from build123d import *
from build123d.topology import SkipClean

# Parameters (mm, degrees)
SKETCH1_R            = 50.8
SKETCH1_W            = 25.4
SKETCH1_H            = 31.75
BOSS_EXTRUDE3_DEPTH  = 50.8
SKETCH2_R            = 50.8
BOSS_EXTRUDE4_DEPTH  = 27.94
SKETCH3_R            = 50.8
BOSS_EXTRUDE5_DEPTH  = 50.8
SKETCH4_R            = 50.8
BOSS_EXTRUDE6_DEPTH  = 27.94
SKETCH5_R            = 50.8
SKETCH5_W            = 25.4
SKETCH5_H            = 31.75
BOSS_EXTRUDE7_DEPTH  = 27.94
BOSS_EXTRUDE8_START  = 27.94
SKETCH6_R            = 50.8
BOSS_EXTRUDE8_DEPTH  = 27.94
BOSS_EXTRUDE9_START  = 50.8
SKETCH7_R            = 50.8
SKETCH7_W            = 31.75
SKETCH7_H            = 25.4
BOSS_EXTRUDE9_DEPTH  = 50.8
BOSS_EXTRUDE10_START = 27.94
SKETCH8_R            = 50.8
BOSS_EXTRUDE10_DEPTH = 27.94
BOSS_EXTRUDE11_START = 27.94
SKETCH9_R            = 50.8
SKETCH9_W            = 25.4
SKETCH9_H            = 31.75
BOSS_EXTRUDE11_DEPTH = 27.94
SKETCH10_R           = 50.8
BOSS_EXTRUDE12_DEPTH = 8.89
BOSS_EXTRUDE13_START = 8.89
SKETCH11_R           = 50.8
BOSS_EXTRUDE13_DEPTH = 8.89
SKETCH12_R           = 25.4
BOSS_EXTRUDE14_DEPTH = 8.89
BOSS_EXTRUDE15_START = 8.89
SKETCH13_R           = 25.4
BOSS_EXTRUDE15_DEPTH = 8.89
SKETCH14_R           = 5
CUT_EXTRUDE1_DEPTH   = 369.166294367
CHAMFER3_SIZE        = 8.89


with BuildPart() as part:
    # Sketch1 → Boss-Extrude3 (new body)
    with BuildSketch(Plane(origin=(0, 0, 0), x_dir=(0, 0, -1), z_dir=(1, 0, 0))):
        Circle(SKETCH1_R)
        with Locations((0, 50.8)):
            Rectangle(SKETCH1_W, SKETCH1_H)
        Polygon((51.392243797, 44.336022628), (23.895937227, 28.461022628), (36.595937227, 6.463977372), (64.092243797, 22.338977372), align=None)
        Polygon((64.092243797, -22.338977372), (36.595937227, -6.463977372), (23.895937227, -28.461022628), (51.392243797, -44.336022628), align=None)
        with Locations((0, -50.8)):
            Rectangle(SKETCH1_W, SKETCH1_H)
        Polygon((-51.392243797, -44.336022628), (-23.895937227, -28.461022628), (-36.595937227, -6.463977372), (-64.092243797, -22.338977372), align=None)
        Polygon((-64.092243797, 22.338977372), (-36.595937227, 6.463977372), (-23.895937227, 28.461022628), (-51.392243797, 44.336022628), align=None)
    extrude(amount=BOSS_EXTRUDE3_DEPTH)

    # Sketch2 → Boss-Extrude4 (add)
    with BuildSketch(Plane(origin=(50.8, 0, 0), x_dir=(0, 0, -1), z_dir=(1, 0, 0))):
        with Locations(Location((0, 0, 0), (0, 0, 164.477512186))):
            Circle(SKETCH2_R)
    extrude(amount=BOSS_EXTRUDE4_DEPTH)

    # Sketch3 → Boss-Extrude5 (add)
    with BuildSketch(Plane(origin=(78.74, 0, 0), x_dir=(0, 0, -1), z_dir=(1, 0, 0))):
        with Locations(Location((0, 0, 0), (0, 0, 165.522487814))):
            Circle(SKETCH3_R)
        Polygon((36.437276545, 12.7), (36.437276545, 0), (36.437276545, -12.7), (68.187276545, -12.7), (68.187276545, 12.7), align=None)
        Polygon((18.218638272, 31.555607132), (29.2171609, 25.205607132), (45.0921609, 52.701913703), (23.095115644, 65.401913703), (7.220115644, 37.905607132), align=None)
        Polygon((29.2171609, -25.205607132), (18.218638272, -31.555607132), (7.220115644, -37.905607132), (23.095115644, -65.401913703), (45.0921609, -52.701913703), align=None)
        Polygon((-7.220115644, -37.905607132), (-18.218638272, -31.555607132), (-29.2171609, -25.205607132), (-45.0921609, -52.701913703), (-23.095115644, -65.401913703), align=None)
        Polygon((-36.437276545, -12.7), (-36.437276545, 0), (-36.437276545, 12.7), (-68.187276545, 12.7), (-68.187276545, -12.7), align=None)
        Polygon((-29.2171609, 25.205607132), (-18.218638272, 31.555607132), (-7.220115644, 37.905607132), (-23.095115644, 65.401913703), (-45.0921609, 52.701913703), align=None)
    extrude(amount=BOSS_EXTRUDE5_DEPTH)

    # Sketch4 → Boss-Extrude6 (add)
    with BuildSketch(Plane(origin=(129.54, 0, 0), x_dir=(0, 0, -1), z_dir=(1, 0, 0))):
        with Locations(Location((0, 0, 0), (0, 0, 164.477512186))):
            Circle(SKETCH4_R)
    extrude(amount=BOSS_EXTRUDE6_DEPTH)

    # Sketch5 → Boss-Extrude7 (add)
    with BuildSketch(Plane(origin=(157.48, 0, 0), x_dir=(0, 0, -1), z_dir=(1, 0, 0))):
        with Locations(Location((0, 0, 0), (0, 0, 164.477512186))):
            Circle(SKETCH5_R)
        with Locations((0, 50.8)):
            Rectangle(SKETCH5_W, SKETCH5_H)
        Polygon((51.392243797, 44.336022628), (23.895937227, 28.461022628), (36.595937227, 6.463977372), (64.092243797, 22.338977372), align=None)
        Polygon((64.092243797, -22.338977372), (36.595937227, -6.463977372), (23.895937227, -28.461022628), (51.392243797, -44.336022628), align=None)
        with Locations((0, -50.8)):
            Rectangle(SKETCH5_W, SKETCH5_H)
        Polygon((-51.392243797, -44.336022628), (-23.895937227, -28.461022628), (-36.595937227, -6.463977372), (-64.092243797, -22.338977372), align=None)
        Polygon((-64.092243797, 22.338977372), (-36.595937227, 6.463977372), (-23.895937227, 28.461022628), (-51.392243797, 44.336022628), align=None)
    extrude(amount=BOSS_EXTRUDE7_DEPTH)

    # Sketch6 → Boss-Extrude8 (add)
    with SkipClean():  # the faces are left unmerged after this step: merging them gives an invalid solid
        with BuildSketch(Plane.ZY.offset(BOSS_EXTRUDE8_START)):
            Circle(SKETCH6_R)
        extrude(amount=-BOSS_EXTRUDE8_DEPTH)

    # Sketch7 → Boss-Extrude9 (add)
    with SkipClean():  # the faces are left unmerged after this step: merging them gives an invalid solid
        with BuildSketch(Plane.ZY.offset(27.94).offset(BOSS_EXTRUDE9_START)):
            with Locations(Location((0, 0, 0), (0, 0, 345.522487814))):
                Circle(SKETCH7_R)
            Polygon((23.095115644, 65.401913703), (45.0921609, 52.701913703), (29.2171609, 25.205607132), (7.220115644, 37.905607132), align=None)
            with Locations((52.312276545, 0)):
                Rectangle(SKETCH7_W, SKETCH7_H)
            Polygon((29.2171609, -25.205607132), (45.0921609, -52.701913703), (23.095115644, -65.401913703), (7.220115644, -37.905607132), align=None)
            Polygon((-7.220115644, -37.905607132), (-23.095115644, -65.401913703), (-45.0921609, -52.701913703), (-29.2171609, -25.205607132), align=None)
            with Locations((-52.312276545, 0)):
                Rectangle(SKETCH7_W, SKETCH7_H)
            Polygon((-29.2171609, 25.205607132), (-45.0921609, 52.701913703), (-23.095115644, 65.401913703), (-7.220115644, 37.905607132), align=None)
        extrude(amount=-BOSS_EXTRUDE9_DEPTH)

    # Sketch8 → Boss-Extrude10 (add)
    with SkipClean():  # the faces are left unmerged after this step: merging them gives an invalid solid
        with BuildSketch(Plane.ZY.offset(78.74).offset(BOSS_EXTRUDE10_START)):
            Circle(SKETCH8_R)
        extrude(amount=-BOSS_EXTRUDE10_DEPTH)

    # Sketch9 → Boss-Extrude11 (add)
    with SkipClean():  # the faces are left unmerged after this step: merging them gives an invalid solid
        with BuildSketch(Plane.ZY.offset(106.68).offset(BOSS_EXTRUDE11_START)):
            with Locations(Location((0, 0, 0), (0, 0, 15.522487814))):
                Circle(SKETCH9_R)
            with Locations((0, 50.8)):
                Rectangle(SKETCH9_W, SKETCH9_H)
            Polygon((51.392243797, 44.336022628), (23.895937227, 28.461022628), (36.595937227, 6.463977372), (64.092243797, 22.338977372), align=None)
            Polygon((64.092243797, -22.338977372), (36.595937227, -6.463977372), (23.895937227, -28.461022628), (51.392243797, -44.336022628), align=None)
            with Locations((0, -50.8)):
                Rectangle(SKETCH9_W, SKETCH9_H)
            Polygon((-51.392243797, -44.336022628), (-23.895937227, -28.461022628), (-36.595937227, -6.463977372), (-64.092243797, -22.338977372), align=None)
            Polygon((-64.092243797, 22.338977372), (-36.595937227, 6.463977372), (-23.895937227, 28.461022628), (-51.392243797, 44.336022628), align=None)
        extrude(amount=-BOSS_EXTRUDE11_DEPTH)

    # Sketch10 → Boss-Extrude12 (add)
    with SkipClean():  # the faces are left unmerged after this step: merging them gives an invalid solid
        with BuildSketch(Plane(origin=(185.42, 0, 0), x_dir=(0, 0, -1), z_dir=(1, 0, 0))):
            with Locations(Location((0, 0, 0), (0, 0, 195.522487814))):
                Circle(SKETCH10_R)
        extrude(amount=BOSS_EXTRUDE12_DEPTH)

    # Sketch11 → Boss-Extrude13 (add)
    with SkipClean():  # the faces are left unmerged after this step: merging them gives an invalid solid
        with BuildSketch(Plane.ZY.offset(134.62).offset(BOSS_EXTRUDE13_START)):
            Circle(SKETCH11_R)
        extrude(amount=-BOSS_EXTRUDE13_DEPTH)

    # Sketch12 → Boss-Extrude14 (add)
    with SkipClean():  # the faces are left unmerged after this step: merging them gives an invalid solid
        with BuildSketch(Plane(origin=(194.31, 0, 0), x_dir=(0, 0, -1), z_dir=(1, 0, 0))):
            Circle(SKETCH12_R)
        extrude(amount=BOSS_EXTRUDE14_DEPTH)

    # Sketch13 → Boss-Extrude15 (add)
    with SkipClean():  # the faces are left unmerged after this step: merging them gives an invalid solid
        with BuildSketch(Plane.ZY.offset(143.51).offset(BOSS_EXTRUDE15_START)):
            with Locations(Location((0, 0, 0), (0, 0, 180))):
                Circle(SKETCH13_R)
        extrude(amount=-BOSS_EXTRUDE15_DEPTH)

    # Sketch14 → Cut-Extrude1 (cut, through all)
    with SkipClean():  # the faces are left unmerged after this step: merging them gives an invalid solid
        with BuildSketch(Plane.ZY.offset(152.4)):
            Circle(SKETCH14_R)
        extrude(amount=-CUT_EXTRUDE1_DEPTH, mode=Mode.SUBTRACT)

    # Chamfer3
    chamfer3_edges = [part.edges().sort_by_distance(p)[0] for p in [
        (194.31, 0, 25.4),
        (-143.51, 0, 25.4),
    ]]
    chamfer(chamfer3_edges, length=CHAMFER3_SIZE - 0.0001)  # a hair under: the kernel refuses the full size


solid = part.part
Input: part model. Units: mm. Frame: model coordinates. A direction names the side the tool comes from. Coordinates: 2 decimals unless noted, no trailing zeros. Order: outer loops, then holes, each group sorted by start corner. A loop starts at its lowest first (then second) coordinate and runs counter-clockwise, first axis right, second up. Notation, with made-up numbers: M 74,11.25 L 114,11.25 A14 ccw 114,21.25 Z; hole C -33,74 d11. An arc over 180 degrees is marked long. Write item = value, one per line. Start each with the question number.
(1) First-contact query: P1, Ø1.5, axis at y = 25.5, z = 1.5, coming from the -X side; P2, Ø5, axis at x = 38, y = -31, coming from the +Z side; P3, Ø5.5, axis at y = 3, z = 58.5, coming from the +X side; P4, Ø1.5, axis at x = 51.5, y = 46.5, coming from the +Z side. Flat tips, straight axial feed; report the tip coordinate or a pass-through.
(2) Reachability of faces 1 (the flat face through (104, -12.7, 59)), 2 (the flat face through (104, -12.7, -59)), 3 (the flat face through (194.31, 29, 19)), 4 (the flat face through (0, 29, -50)) from +Z, -Z, +X, -X, +Y, -Y: full face, straight path, thin tool, end or side. Return the list, or none.
(3) Pull-direction query (Y, two-part tool) for faces 5 (the flat face through (25.04, -18.03, -56.63)), 6 (the flat face through (185.42, -29, 50)), 7 (the flat face through (25, -66.675, 0)); classes: released by +Y, released by -Y, zero draft, split by the parting line, or undercut.
(4) Section B-B on x = -62. Output: boundary loops of the cut face in (y, z).
(5) Section C-C on y = -40. Give the number of separate pieces and of enclosed holes in the cut face, and give its area (3 significant figures).
(6) Line query: line 1 along X through (y, z) = (-39, 52); line 2 along Y through (x, z) = (121.5, 0); line 3 along Y through (x, z) = (46, 0) (3 decimals). Output: solid intervals per line, ascending. Write a range as [from, to].
(7) Section D-D on x = 62. Output: boundary loops of the cut face in (y, z).
(8) Section A-A on x = 4. Output: boundary loops of the cut face in (y, z) (3 decimals).
Result set:
q1.P1 = -152.4
q1.P2 = 60.54
q1.P3 = 129.54
q1.P4 = 22.08
q2.face_1 = +Z, +X, -X, -Y
q2.face_2 = -Z, +X, -X, -Y
q2.face_3 = +X
q2.face_4 = -Z, +Y
q3.face_5 = undercut
q3.face_6 = zero draft
q3.face_7 = released by -Y
q4.outline = M -65.4,-23.1 L -52.7,-45.09 L -36.25,-35.59 A50.8 ccw -12.7,-49.19 L -12.7,-68.19 L 12.7,-68.19 L 12.7,-49.19 A50.8 ccw 36.25,-35.59 L 52.7,-45.09 L 65.4,-23.1 L 48.95,-13.59 A50.8 ccw 48.95,13.59 L 65.4,23.1 L 52.7,45.09 L 36.25,35.59 A50.8 ccw 12.7,49.19 L 12.7,68.19 L -12.7,68.19 L -12.7,49.19 A50.8 ccw -36.25,35.59 L -52.7,45.09 L -65.4,23.1 L -48.95,13.59 A50.8 ccw -48.95,-13.59 Z; hole C 0,0 d10
q5.separate_pieces = 7
q5.enclosed_holes = 0
q5.area = 24,600 mm²
q6.line_1 = [-134.62, -106.68], [0, 50.8], [157.48, 185.42]
q6.line_2 = [-50.8, -5], [5, 50.8]
q6.line_3 = [-66.675, -5], [5, 66.675]
q7.outline = C 0,0 d101.6; hole C 0,0 d10
q8.outline = M -66.675,-12.7 L -49.187,-12.7 A50.8 ccw -35.592,-36.247 L -44.336,-51.392 L -22.339,-64.092 L -13.595,-48.947 A50.8 ccw 13.595,-48.947 L 22.339,-64.092 L 44.336,-51.392 L 35.592,-36.247 A50.8 ccw 49.187,-12.7 L 66.675,-12.7 L 66.675,12.7 L 49.187,12.7 A50.8 ccw 35.592,36.247 L 44.336,51.392 L 22.339,64.092 L 13.595,48.947 A50.8 ccw -13.595,48.947 L -22.339,64.092 L -44.336,51.392 L -35.592,36.247 A50.8 ccw -49.187,12.7 L -66.675,12.7 Z; hole C 0,0 d10
